Design review of the part built by this model. Coordinates are the model's own, in mm. A direction names the side the tool comes from. Coordinates: 2 decimals unless noted, no trailing zeros. Order: outer loops, then holes, each group sorted by start corner. A loop starts at its lowest first (then second) coordinate and runs counter-clockwise, first axis right, second up. Notation, with made-up numbers: M 23.5,53 L 81.5,53 A18 cw 81.5,77 Z; hole C 45,52.25 d1. An arc over 180 degrees is marked long. Answer as a JSON object with one key per item and string values.
from build123d import *

# Parameters (mm, degrees)
SKETCH_R        = 2.3622
SKETCH_R_2      = 4.7625
PAD_DEPTH       = 3.175
FILLET_R        = 6.35
FILLET001_R     = 6.35
FILLET002_R     = 6.35
FILLET003_R     = 6.35
FILLET004_R     = 6.35
FILLET005_R     = 3.175
FILLET006_R     = 3.175
FILLET007_R     = 6.35
FILLET008_R     = 6.35
FILLET009_R     = 6.35
FILLET010_R     = 6.35
FILLET011_R     = 6.35
FILLET012_R     = 3.175
FILLET013_R     = 3.175
SKETCH001_R     = 1.651
POCKET_DEPTH    = 3.176
SKETCH002_R     = 2.2479
POCKET001_DEPTH = 3.176
SKETCH003_R     = 2.2479
POCKET002_DEPTH = 4.99999


with BuildPart() as part:
    # Sketch → Pad (new body)
    with BuildSketch(Plane(origin=(-14.3421, 44.2432, 43.6758), x_dir=(1, 0, 0), z_dir=(0, 0, 1))):
        Polygon((40.4368, 35.9029), (-40.4368, 35.9029), (-40.4368, 88.9), (-59.4868, 88.9), (-127.8382, 12.7), (-127.8382, -12.7), (-59.4868, -88.9), (-40.4368, -88.9), (-40.4368, -35.9029), (40.4368, -35.9029), (40.4368, -88.9), (62.6618, -88.9), (62.6618, 88.9), (40.4368, 88.9), align=None)
        with Locations((-21.3868, 29.5529)):
            Circle(SKETCH_R, mode=Mode.SUBTRACT)
        with Locations((-21.3868, 16.8529)):
            Circle(SKETCH_R, mode=Mode.SUBTRACT)
        with Locations((-21.3868, -16.8529)):
            Circle(SKETCH_R, mode=Mode.SUBTRACT)
        with Locations((-21.3868, -29.5529)):
            Circle(SKETCH_R, mode=Mode.SUBTRACT)
        with Locations((15.0368, 29.5529)):
            Circle(SKETCH_R, mode=Mode.SUBTRACT)
        with Locations((15.24, 16.8529)):
            Circle(SKETCH_R, mode=Mode.SUBTRACT)
        with Locations((15.24, -16.8529)):
            Circle(SKETCH_R, mode=Mode.SUBTRACT)
        with Locations((15.24, -29.5529)):
            Circle(SKETCH_R, mode=Mode.SUBTRACT)
        with Locations((-115.1382, 0)):
            Circle(SKETCH_R_2, mode=Mode.SUBTRACT)
    extrude(amount=PAD_DEPTH)

    # Fillet
    fillet_edges = [part.edges().sort_by_distance(p)[0] for p in [
        (-142.1803, 31.5432, 45.2633),
    ]]
    fillet(fillet_edges, radius=FILLET_R)

    # Fillet001
    fillet001_edges = [part.edges().sort_by_distance(p)[0] for p in [
        (-73.8289, -44.6568, 45.2633),
    ]]
    fillet(fillet001_edges, radius=FILLET001_R)

    # Fillet002
    fillet002_edges = [part.edges().sort_by_distance(p)[0] for p in [
        (-54.7789, -44.6568, 45.2633),
    ]]
    fillet(fillet002_edges, radius=FILLET002_R)

    # Fillet003
    fillet003_edges = [part.edges().sort_by_distance(p)[0] for p in [
        (-54.7789, 8.3403, 45.2633),
    ]]
    fillet(fillet003_edges, radius=FILLET003_R)

    # Fillet004
    fillet004_edges = [part.edges().sort_by_distance(p)[0] for p in [
        (26.0947, 8.3403, 45.2633),
    ]]
    fillet(fillet004_edges, radius=FILLET004_R)

    # Fillet005
    fillet005_edges = [part.edges().sort_by_distance(p)[0] for p in [
        (26.0947, -44.6568, 45.2633),
    ]]
    fillet(fillet005_edges, radius=FILLET005_R)

    # Fillet006
    fillet006_edges = [part.edges().sort_by_distance(p)[0] for p in [
        (48.3197, -44.6568, 45.2633),
    ]]
    fillet(fillet006_edges, radius=FILLET006_R)

    # Fillet007
    fillet007_edges = [part.edges().sort_by_distance(p)[0] for p in [
        (-142.1803, 56.9432, 45.2633),
    ]]
    fillet(fillet007_edges, radius=FILLET007_R)

    # Fillet008
    fillet008_edges = [part.edges().sort_by_distance(p)[0] for p in [
        (-73.8289, 133.1432, 45.2633),
    ]]
    fillet(fillet008_edges, radius=FILLET008_R)

    # Fillet009
    fillet009_edges = [part.edges().sort_by_distance(p)[0] for p in [
        (-54.7789, 133.1432, 45.2633),
    ]]
    fillet(fillet009_edges, radius=FILLET009_R)

    # Fillet010
    fillet010_edges = [part.edges().sort_by_distance(p)[0] for p in [
        (26.0947, 80.1461, 45.2633),
    ]]
    fillet(fillet010_edges, radius=FILLET010_R)

    # Fillet011
    fillet011_edges = [part.edges().sort_by_distance(p)[0] for p in [
        (-54.7789, 80.1461, 45.2633),
    ]]
    fillet(fillet011_edges, radius=FILLET011_R)

    # Fillet012
    fillet012_edges = [part.edges().sort_by_distance(p)[0] for p in [
        (26.0947, 133.1432, 45.2633),
    ]]
    fillet(fillet012_edges, radius=FILLET012_R)

    # Fillet013
    fillet013_edges = [part.edges().sort_by_distance(p)[0] for p in [
        (48.3197, 133.1432, 45.2633),
    ]]
    fillet(fillet013_edges, radius=FILLET013_R)

    # Sketch001 → Pocket (cut, through all)
    with BuildSketch(Plane(origin=(-14.3421, 44.2432, 46.8508), x_dir=(1, 0, 0), z_dir=(0, 0, 1))):
        with Locations((-56.906653, 47.390231)):
            Circle(SKETCH001_R)
        with Locations((-65.098153, 47.390231)):
            Circle(SKETCH001_R)
        with Locations((-56.906653, 56.915231)):
            Circle(SKETCH001_R)
        with Locations((-48.715153, 47.390231)):
            Circle(SKETCH001_R)
        with Locations((-56.906653, 37.865231)):
            Circle(SKETCH001_R)
    extrude(amount=-POCKET_DEPTH, mode=Mode.SUBTRACT)

    # Sketch002 → Pocket001 (cut, through all)
    with BuildSketch(Plane(origin=(-14.3421, 44.2432, 46.8508), x_dir=(1, 0, 0), z_dir=(0, 0, 1))):
        with Locations((-85.394727, -52.884764)):
            Circle(SKETCH002_R)
        with Locations((-64.1943, -76.519577)):
            Circle(SKETCH002_R)
        with Locations((-64.1943, 76.519577)):
            Circle(SKETCH002_R)
        with Locations((-85.394727, 52.884764)):
            Circle(SKETCH002_R)
    extrude(amount=-POCKET001_DEPTH, mode=Mode.SUBTRACT)

    # Sketch003 → Pocket002 (cut)
    with BuildSketch(Plane(origin=(-14.3421, 44.2432, 46.8508), x_dir=(1, 0, 0), z_dir=(0, 0, 1))):
        with Locations((57.8993, -79.375)):
            Circle(SKETCH003_R)
        with Locations((57.8993, -28.575)):
            Circle(SKETCH003_R)
        with Locations((57.8993, 79.375)):
            Circle(SKETCH003_R)
        with Locations((57.8993, 28.575)):
            Circle(SKETCH003_R)
    extrude(amount=-POCKET002_DEPTH, mode=Mode.SUBTRACT)


solid = part.part
1) Insertion check: pin 1 Ø6 at (x, y) = (43.56, -35.13) entering from -Z; pin 2 Ø1.5 at (x, z) = (-106, 44.5) entering from +Y; pin 3 Ø1 at (x, z) = (-9, 45) entering from +Y. Each pin has a flat end and moves straight along its axis. Give the tip position at first contact, or say it passes through.
Taken from the geometry:
{"pin 1": "stops at z = 43.68", "pin 2": "stops at y = 98.11", "pin 3": "stops at y = 80.15"}
2) To check wall thickness, follow L1, parallel to Y at x = -100, z = 44.35; L2, parallel to X at y = 74.5, z = 44.4; L3, parallel to X at y = 81, z = 45.5. State the ranges of each line that lie inside material, in increasing order.
Taken from the geometry:
{"L1": "y = -15.48 to -10.87, -6.41 to 94.9, 99.36 to 103.97", "L2": "x = -126.43 to -37.98, -33.47 to -1.56, 2.95 to 42.07, 45.05 to 48.32", "L3": "x = -120.6 to -72.47, -70.03 to -51.61, 22.93 to 48.32"}
3) Add section B-B (x = -29.5). State the section outline as (y, z) points, and give its area (3 significant figures).
Taken from the geometry:
{"outline": "M 8.34,43.68 L 80.15,43.68 L 80.15,46.85 L 8.34,46.85 Z", "area": "228 mm2"}
4) Add section A-A (y = 111). State the section outline as (x, z) points.
Taken from the geometry:
{"outline": "M -93.69,43.68 L -54.78,43.68 L -54.78,46.85 L -93.69,46.85 Z; M 26.09,43.68 L 48.32,43.68 L 48.32,46.85 L 26.09,46.85 Z"}
5) Add section C-C (z = 46.25). Count the separate pieces of the cut face and the enclosed holes in it, and give its area (3 significant figures).
Taken from the geometry:
{"separate pieces": "1", "enclosed holes": "22", "area": "19,700 mm2"}
6) Mouldability with a two-part tool opening along X and no side actions: class faces 4 (the cylindrical face through (0.386, 12.384, 45.241)), 5 (the cylindrical face through (-98.7, 95.134, 45.286)), 6 (the flat face through (-108.593, -5.901, 45.241)) as released by +X, released by -X, zero draft, split by the parting line, or undercut.
Taken from the geometry:
{"face 4": "undercut", "face 5": "undercut", "face 6": "released by -X"}
7) Add section D-D (x = -116). State the section outline as (y, z) points.
Taken from the geometry:
{"outline": "M 2.36,43.68 L 86.13,43.68 L 86.13,46.85 L 2.36,46.85 Z"}
8) Tool access review of faces 1 (the cylindrical face through (1.78, 71.7, 45.24)), 2 (the cylindrical face through (-56.688, 131.332, 45.286)), 3 (the cylindrical face through (-56.69, -42.85, 45.29)): name each direction out of +Z, -Z, +X, -X, +Y, -Y from which nothing blocks a thin tool from reaching the whole face with its end or side.
Taken from the geometry:
{"face 1": "+Z, -Z", "face 2": "+Z, -Z, +Y", "face 3": "+Z, -Z, -Y"}
